Design review of the part built by this model. Coordinates are the model's own, in mm. Round coordinates to 2 decimals unless told otherwise and drop trailing zeros. Order: outer loops, then holes, each group sorted by start corner. A loop starts at its lowest first (then second) coordinate and runs counter-clockwise, first axis right, second up. Notation, with made-up numbers: M -33.5,76 L -26.5,76 A12 cw -26.5,84 Z; hole C -32,31.5 d9. An arc over 180 degrees is marked long. Write each question's results on one line, items separated by ' | '. Start each with the question number.
Item 1: Wall thickness on line 1 (X direction, y = 3, z = 47); line 2 (X direction, y = 9, z = 12.5) (3 decimals); line 3 (Y direction, x = 22, z = 36): over which ranges is each line inside the solid? List them lowest first. Write a range as [from, to].
Item 2: Take a section at C-C, the plane y = 16.5. Write out the cut boundary in (x, z).
Item 3: Take a section at B-B, the plane z = 22. Write out the cut boundary in (x, y).
Item 4: The part is to be moulded in two halves that separate along X. For faces 1 (the flat face through (11, 13, 94.146)), 2 (the flat face through (-21.838, 12, 46)), 3 (the cylindrical face through (4.916, 3.004, 46.414)), 4 (the flat face through (64.737, 12, 37)), say which applies: +X half, -X half, draft (parallel to the pull), parting line (faces both ways), or undercut.
Item 5: Take a section at D-D, the plane x = 59.5. Write out the cut boundary in (y, z), plus the area to 3 significant figures.
Item 6: Take a section at A-A, the plane y = 0. Write out the cut boundary in (x, z), plus the area to 3 significant figures.
Item 7: Clearance check with a flat-ended pin moving along its axis: pin 1 (18 mm diameter, centred on x = 14.45, y = 0, fed in from +Z). State where the tip first meets the part, or that it passes through.
```python
from build123d import *

# Parameters (mm, degrees)
F0_W     = 86.574215
F0_H     = 83.982148
F1_DEPTH = 94.14638
F2_SIZE  = 20
F4_D     = 20


with BuildPart() as f1:
    # F0 (on Top) → F1 (new body)
    with BuildSketch(Plane.XY):
        with Locations((21.449423, 12.660671)):
            Rectangle(F0_W, F0_H)
    extrude(amount=F1_DEPTH)

    # F2
    f2_edges = [f1.edges().sort_by_distance(p)[0] for p in [
        (64.73653, 12.660671, 94.14638),
    ]]
    chamfer(f2_edges, length=F2_SIZE)

    # F4 (through all)
    with Locations(Plane.XY.offset(94.14638)):
        with Locations((14.453897, 0)):
            Hole(F4_D / 2)


solid = f1.part
```
Results list:
1) line 1: [-21.84, 4.91], [23.99, 64.74] | line 2: [-21.838, 10.095], [18.813, 64.737] | line 3: [-29.33, -6.56], [6.56, 54.65]
2) outline: M -21.84,0 L 64.74,0 L 64.74,74.15 L 44.74,94.15 L -21.84,94.15 Z
3) outline: M -21.84,-29.33 L 64.74,-29.33 L 64.74,54.65 L -21.84,54.65 Z; hole C 14.45,0 d20
4) face 1: draft | face 2: -X half | face 3: undercut | face 4: +X half
5) outline: M -29.33,0 L 54.65,0 L 54.65,79.38 L -29.33,79.38 Z | area: 6,670 mm²
6) outline: M -21.84,0 L 4.45,0 L 4.45,94.15 L -21.84,94.15 Z; M 24.45,0 L 64.74,0 L 64.74,74.15 L 44.74,94.15 L 24.45,94.15 Z | area: 6,070 mm²
7) pin 1: through
